Work out the finished part from the listing and answer in its coordinate system (mm). Coordinates: 2 decimals unless noted, no trailing zeros. Loops run counter-clockwise (first coordinate to the right, second up) from the corner with the lowest first, then second, coordinate; pieces in that order, holes last. Notation, with made-up numbers: (64, 16) -> (121, 16) arc R7 cw to (121, 27) -> close; hole circle Ø5 at (-14.5, -4). An arc over 180 degrees is marked (long way). One line per question, with ' | ' between items.
```python
from build123d import *

# Parameters (mm, degrees)
SKETCH1_R           = 7.5
BOSS_EXTRUDE1_DEPTH = 70
SCALE1_SCALE        = 10
SCALE2_SCALE        = 0.75


with BuildPart() as part:
    # Sketch1 → Boss-Extrude1 (new body)
    with BuildSketch(Plane(origin=(0, 0, 0), x_dir=(1, 0, 0), z_dir=(0, 1, 0))):
        Circle(SKETCH1_R)
    extrude(amount=BOSS_EXTRUDE1_DEPTH)


with BuildPart() as part_1:
    # Scale1: scaled about (0, 0, 0)
    add(part.part.scale(SCALE1_SCALE))


with BuildPart() as part_2:
    # Scale2: scaled about (0, 350, 0)
    add(part_1.part.scale(SCALE2_SCALE).moved(Location((0, 87.5, 0))))


solid = part_2.part
```
1) Find the intervals of material crossed by line 1 along Z through (x, y) = (3, 474); line 2 along Z through (x, y) = (-44, 551); line 3 along X through (y, z) = (472, 42.5), in increasing order.
Check values:
line 1: z = -56.17 to 56.17 | line 2: z = -35.04 to 35.04 | line 3: x = -36.85 to 36.85
2) Find section A-A (y = 421). Write down the section's boundary in (x, z).
Check values:
outline: circle Ø112.5 at (0, 0)
3) Find section B-B (x = -28). Write down the section's boundary in (y, z).
Check values:
outline: (87.5, -48.79) -> (612.5, -48.79) -> (612.5, 48.79) -> (87.5, 48.79) -> close
4) Find section C-C (z = -46). Write down the section's boundary in (x, y), plus the area to 3 significant figures.
Check values:
outline: (-32.37, 87.5) -> (32.37, 87.5) -> (32.37, 612.5) -> (-32.37, 612.5) -> close | area: 34,000 mm^2
5) Flat-ended cylindrical pins translate along their axes: pin 1 (3 mm diameter, centred on x = -5.5, y = 556, fed in from +Z); pin 2 (1 mm diameter, centred on x = 9.5, y = 525.5, fed in from +Z); pin 3 (1.5 mm diameter, centred on y = 255.5, z = 11.5, fed in from -X). Find the tip coordinate at first contact, or state that the pin passes through.
Check values:
pin 1: stops at z = 56.11 | pin 2: stops at z = 55.53 | pin 3: stops at x = -55.21
